Geometry check sheet. Reference: the model listing, model coordinates, mm. Face numbers are marked on the shaded views. A direction names the side the tool comes from. Give positions to 0.01 mm unless a question says otherwise; leave off trailing zeros. Order: outer loops, then holes, each group sorted by start corner. A loop starts at its lowest first (then second) coordinate and runs counter-clockwise, first axis right, second up. Notation, with made-up numbers: M -18,3.25 L 35,3.25 A35 ccw 35,41.25 Z; hole C 11.25,-28.5 d8. An arc over 180 degrees is marked long. Answer as CSV lines item,"result". Start each with the question number.
Q1. Section check D-D, the plane y = -7.5. Count the separate pieces of the cut face and the enclosed holes in it, then the cut area to 3 significant figures.
Q2. Section check C-C, the plane z = 5. Record the boundary of the cut face in (x, y), then the cut area to 3 significant figures.
Q3. Section check A-A, the plane z = 47.5. Record the boundary of the cut face in (x, y), then the cut area to 3 significant figures.
Q4. Set-up check for the marked faces 1, 2 and 3: record each of +Z, -Z, +X, -X, +Y, -Y from which the full face is reachable in a straight line by a thin tool's end or side.
Q5. Thickness scan on line 1 (X direction, y = -6, z = 64); line 2 (Z direction, x = 12, y = -2.75); line 3 (Z direction, x = 3.5, y = -2). Record the ranges inside material, lowest first.
Q6. Mould release check, pull along Z, two halves, no side actions. Record for the marked faces 4, 5 and 6: +Z half, -Z half, draft (parallel to the pull), parting line (faces both ways), or undercut.
Q7. Section check B-B, the plane x = 10. Record the boundary of the cut face in (y, z).
Q8. Go/stop test with flat-tipped pins: pin 1 (6 mm diameter, centred on x = 9.5, y = -6.5, fed in from -Z); pin 2 (3.5 mm diameter, centred on y = -3.5, z = 29, fed in from +X); pin 3 (1 mm diameter, centred on y = -2.5, z = 29, fed in from -X). Record where each tip stops, or that it passes through.
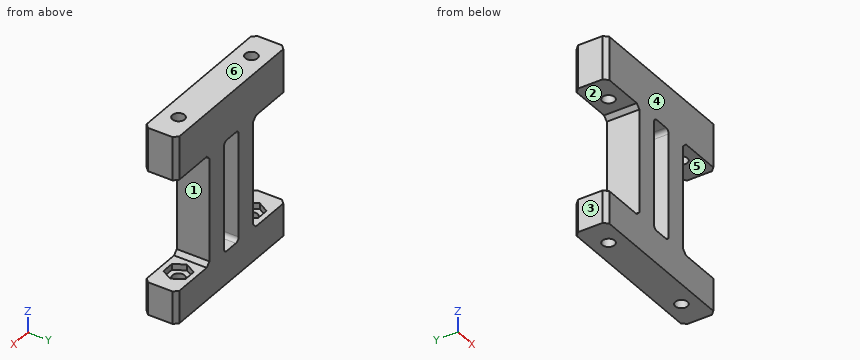
```python
from build123d import *

# Parameters (mm, degrees)
F1_DEPTH  = 12
F2_R      = 2.25
F3_DEPTH  = 16
F4_SIZE   = 1.5
F5_W      = 8
F5_H      = 41
F6_DEPTH  = 12.001
F7_R      = 1.5
F8_R      = 2.25
F9_DEPTH  = 12
F11_DEPTH = 2.2


with BuildPart() as f1:
    # F0 (on Front) → F1 (new body)
    with BuildSketch(Plane.XZ):
        Polygon((0, 12), (0, 0), (60, 0), (60, 12), (42, 12), (42, 53), (60, 53), (60, 69), (0, 69), (0, 53), (18, 53), (18, 12), align=None)
    extrude(amount=F1_DEPTH)

    # F2 (on face) → F3 (cut, through all)
    with BuildSketch(Plane(origin=(0, 0, 53), x_dir=(1, 0, 0), z_dir=(0, 0, -1))):
        with Locations((10, 6)):
            Circle(F2_R)
        with Locations((50, 6)):
            Circle(F2_R)
    extrude(amount=-F3_DEPTH, mode=Mode.SUBTRACT)

    # F4
    f4_edges = [f1.edges().sort_by_distance(p)[0] for p in [
        (60, -12, 61),
        (60, -12, 6),
        (60, 0, 6),
        (60, 0, 61),
        (0, -12, 61),
        (0, 0, 61),
        (0, 0, 6),
        (0, -12, 6),
        (18, -6, 12),
        (18, -6, 53),
        (42, -6, 53),
        (42, -6, 12),
    ]]
    chamfer(f4_edges, length=F4_SIZE)

    # F5 (on face) → F6 (cut, through all)
    with BuildSketch(Plane.XZ.offset(12)):
        with Locations((30, 32.5)):
            Rectangle(F5_W, F5_H)
    extrude(amount=-F6_DEPTH, mode=Mode.SUBTRACT)

    # F7
    f7_edges = [f1.edges().sort_by_distance(p)[0] for p in [
        (26, -6, 53),
        (34, -6, 53),
        (34, -6, 12),
        (26, -6, 12),
    ]]
    fillet(f7_edges, radius=F7_R)

    # F8 (on face) → F9 (cut, through all)
    with BuildSketch(Plane(origin=(0, 0, 0), x_dir=(1, 0, 0), z_dir=(0, 0, -1))):
        with Locations((50, 6)):
            Circle(F8_R)
        with Locations((10, 6)):
            Circle(F8_R)
    extrude(amount=-F9_DEPTH, mode=Mode.SUBTRACT)

    # F10 (on face) → F11 (cut)
    with BuildSketch(Plane.XY.offset(12)):
        Polygon((7.690599, -10), (12.309401, -10), (14.618802, -6), (12.309401, -2), (7.690599, -2), (5.381198, -6), align=None)
        Polygon((52.314719, -9.996925), (54.618798, -5.993857), (52.304079, -1.996932), (47.685281, -2.003075), (45.381202, -6.006143), (47.695921, -10.003068), align=None)
    extrude(amount=-F11_DEPTH, mode=Mode.SUBTRACT)


solid = f1.part
```
Answer block:
1,separate pieces,"5"
1,enclosed holes,"1"
1,area,"2,140 mm2"
2,outline,"M 0,-10.5 L 1.5,-12 L 58.5,-12 L 60,-10.5 L 60,-1.5 L 58.5,0 L 1.5,0 L 0,-1.5 Z; hole C 10,-6 d4.5; hole C 50,-6 d4.5"
2,area,"684 mm2"
3,outline,"M 18,-12 L 26,-12 L 26,0 L 18,0 Z; M 34,-12 L 42,-12 L 42,0 L 34,0 Z"
3,area,"192 mm2"
4,face 1,"+X, +Y, -Y"
4,face 2,"-X, +Y, -Y"
4,face 3,"+Z, -Z, -X, +Y, -Y"
5,line 1,"x = 0 to 7.75, 12.25 to 47.75, 52.25 to 60"
5,line 2,"z = 0 to 9.8, 53 to 69"
5,line 3,"z = 0 to 12, 53 to 69"
6,face 4,"draft"
6,face 5,"undercut"
6,face 6,"+Z half"
7,outline,"M -12,0 L -8.25,0 L -8.25,9.8 L -10,9.8 L -10,12 L -12,12 Z; M -12,53 L -8.25,53 L -8.25,69 L -12,69 Z; M -3.75,0 L 0,0 L 0,12 L -2,12 L -2,9.8 L -3.75,9.8 Z; M -3.75,53 L 0,53 L 0,69 L -3.75,69 Z"
8,pin 1,"stops at z = 0"
8,pin 2,"stops at x = 42"
8,pin 3,"stops at x = 18"
